Autodesk Inventor part; units mm, degrees
ref_plane "YZ Plane" through (0, 0, 0) normal (1, 0, 0) x (0, 1, 0)
ref_plane "XZ Plane" through (0, 0, 0) normal (0, 1, 0) x (-1, 0, 0)
ref_plane "XY Plane" through (0, 0, 0) normal (0, 0, 1) x (1, 0, 0)
sketch "Sketch1" plane through (0, 0, 0) normal (0, 1, 0) x (-1, 0, 0)
  line L0 (0, 0) -> (25, 0)
  line L1 (25, 0) -> (25, -145)
  line L2 (25, -145) -> (0, -145)
  line L3 (0, -145) -> (0, 0)
  dimension "d0" = 25
  dimension "d1" = 145
extrude "Extrusion1" add sketch "Sketch1" along normal blind 2
sketch "Sketch2" plane through (0, 2, 0) normal (0, 1, 0) x (1, 0, 0)
  line L0 (-25, 0) -> (0, 0)
  line L1 (0, 0) -> (0, 145)
  line L2 (0, 145) -> (-25, 145)
  line L3 (-25, 145) -> (-25, 0)
  line L4 (-25, 145) -> (-25, 0)
  line L5 (0, 0) -> (-25, 0)
  line L6 (-25, 0) -> (-25, 2)
  line L7 (-25, 2) -> (0, 2)
  line L8 (0, 2) -> (0, 0)
  line L9 (0, 145) -> (-25, 145)
  line L10 (-25, 145) -> (-25, 143)
  line L11 (-25, 143) -> (0, 143)
  line L12 (0, 143) -> (0, 145)
  dimension "d4" = 2
  dimension "d5" = 2
extrude "Extrusion2" add sketch "Sketch2" along normal blind 20 contours L3 L7 L1 L0 | L3 L2 L1 L11
sketch "Sketch3" plane through (-25, 0, 0) normal (0, 0, 1) x (1, 0, 0)
  line L0 (25, 0) -> (0, 0)
  line L1 (25, 0) -> (25, 22)
  line L2 (0, 22) -> (25, 22)
  line L3 (0, 0) -> (0, 22)
  circle A0 centre (12.5, 11) radius 3.175
  circle A1 centre (16.7687, 11) radius 0.3969
  circle A2 centre (8.2312, 11) radius 0.3969
  dimension "d8" = 12.5
  dimension "d9" = 11
  dimension "d10" = 6.35
  dimension "d15" = 0.7937
  dimension "d16" = 0.7937
  dimension "d17" = 8.2312
  dimension "d19" = 8.2312
  dimension "d20" = 11
  dimension "d21" = 11
extrude "Extrusion4" cut sketch "Sketch3" against normal up to surface (145 mm away) contours A0 | A1 | A2
equation "\"d16\" = d15"
properties part number "motor-rail"
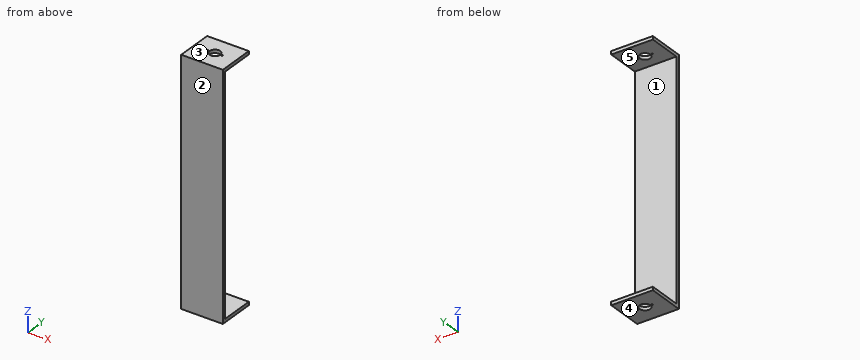
Input: part model. Units: mm. Frame: model coordinates. Face numbers are marked on the shaded views. A direction names the side the tool comes from. Coordinates: 2 decimals unless noted, no trailing zeros. Loops run counter-clockwise (first coordinate to the right, second up) from the corner with the lowest first, then second, coordinate; pieces in that order, holes last. Notation, with made-up numbers: (-11.75, -11.5) -> (22.25, -11.5) arc R15 cw to (22.25, 5.5) -> close; hole circle Ø8 at (-34.5, 78.25). An arc over 180 degrees is marked (long way). Write each question's results on one line, items separated by ' | '. Start each with the question number.
Q1. Section C-C, the plane x = -1.75. Return the cut outline in (y, z), plus the area to 3 significant figures.
Q2. Section B-B, the plane y = 17.25. Return the cut outline in (x, z).
Q3. Section A-A, the plane x = -12.5. Return the cut outline in (y, z) (3 decimals), plus the area to 3 significant figures.
Q4. Pin query (flat end, axial travel): pin 1 (2 mm diameter, centred on x = -9.5, z = -47, fed in from +Y). Return the tip coordinate at first contact, or that it passes through.
Q5. Ray query, line 1 (Z direction, x = -16.5, y = 16.75); line 2 (Y direction, x = -18, z = -71.5). Return the intervals inside material, ascending. Write a range as from..to.
Q6. Pull-direction query (Z, two-part tool) for the marked faces 3, 4 and 5; classes: released by +Z, released by -Z, zero draft, split by the parting line, or undercut.
Q7. Reachability of the marked faces 1 and 2 from +Z, -Z, +X, -X, +Y, -Y: full face, straight path, thin tool, end or side. Return the list, or none.
Q8. Section D-D, the plane z = -118.5. Return the cut outline in (x, y).
Found:
1) outline: (0, -145) -> (22, -145) -> (22, -143) -> (2, -143) -> (2, -2) -> (22, -2) -> (22, 0) -> (0, 0) -> close | area: 370 mm2
2) outline: (-25, -145) -> (0, -145) -> (0, -143) -> (-25, -143) -> close; (-25, -2) -> (0, -2) -> (0, 0) -> (-25, 0) -> close
3) outline: (0, -145) -> (7.825, -145) -> (7.825, -143) -> (2, -143) -> (2, -2) -> (7.825, -2) -> (7.825, 0) -> (0, 0) -> close; (14.175, -145) -> (22, -145) -> (22, -143) -> (14.175, -143) -> close; (14.175, -2) -> (22, -2) -> (22, 0) -> (14.175, 0) -> close | area: 345 mm2
4) pin 1: y = 2
5) line 1: -145..-143, -2..0 | line 2: 0..2
6) face 3: released by +Z | face 4: released by -Z | face 5: undercut
7) face 1: +X, -X, +Y | face 2: +Z, -Z, +X, -X, -Y
8) outline: (-25, 0) -> (0, 0) -> (0, 2) -> (-25, 2) -> close
